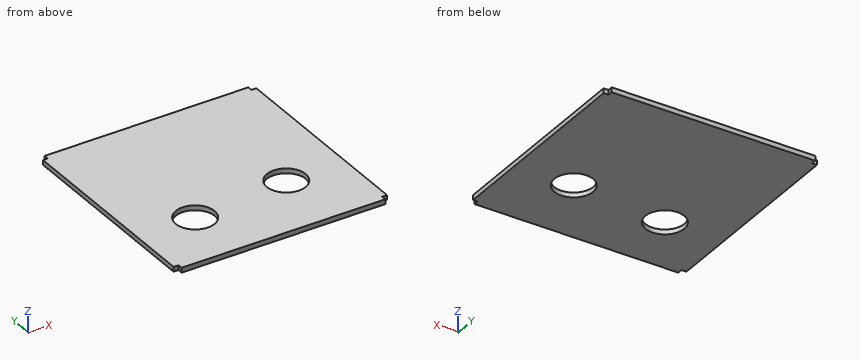
```python
from build123d import *

# Parameters (mm, degrees)
SKETCH1_W           = 279.4
SKETCH1_H           = 279.4
BOSS_EXTRUDE1_DEPTH = 6.35
SKETCH3_R           = 25.4
CUT_EXTRUDE2_DEPTH  = 198.667656687
SKETCH4_W           = 6.35
SKETCH4_H           = 6.35
CUT_EXTRUDE3_DEPTH  = 198.667656687


with BuildPart() as part:
    # Sketch1 → Boss-Extrude1 (new body)
    with BuildSketch(Plane.XY):
        Rectangle(SKETCH1_W, SKETCH1_H)
    extrude(amount=BOSS_EXTRUDE1_DEPTH)

    # Sketch3 → Cut-Extrude2 (cut, through all)
    with BuildSketch(Plane.XY.offset(6.35)):
        with Locations((-63.668986787, -58.7375)):
            Circle(SKETCH3_R)
        with Locations((62.797291543, -47.625)):
            Circle(SKETCH3_R)
    extrude(amount=-CUT_EXTRUDE2_DEPTH, mode=Mode.SUBTRACT)

    # Sketch4 → Cut-Extrude3 (cut, through all)
    with BuildSketch(Plane.XY.offset(6.35)):
        with Locations((-136.525, 136.525)):
            Rectangle(SKETCH4_W, SKETCH4_H)
        with Locations((136.525, 136.525)):
            Rectangle(SKETCH4_W, SKETCH4_H)
        with Locations((136.525, -136.525)):
            Rectangle(SKETCH4_W, SKETCH4_H)
        with Locations((-136.525, -136.525)):
            Rectangle(SKETCH4_W, SKETCH4_H)
    extrude(amount=-CUT_EXTRUDE3_DEPTH, mode=Mode.SUBTRACT)


solid = part.part
```
Part model, mm, in its own coordinate system. Coordinates: 2 decimals unless noted, no trailing zeros. Write each loop counter-clockwise with the first axis right and the second up, starting at its lowest first coordinate (ties: lowest second). Pieces come first, ordered by that corner, then holes.
Item 1: Pin check, flat tips, straight feed: pin 1 (1.9 mm diameter, centred on x = -135, z = 2.5, fed in from +Y); pin 2 (1.9 mm diameter, centred on y = -136, z = 3, fed in from +X); pin 3 (3 mm diameter, centred on y = -136, z = 3, fed in from -X). Stop position of each tip, or through.
Item 2: Probe line 1 (X direction, y = -63.5, z = 5.25); line 2 (X direction, y = -65, z = 3.75); line 3 (X direction, y = -29, z = 3.25). List the from-to ranges inside material, lowest first.
Item 3: Slice it at A-A (x = 52.5). Write the cut outline in (y, z), and give its area (3 significant figures).
Item 4: Slice it at D-D (x = -85). Write the cut outline in (y, z), and give its area (3 significant figures).
Item 5: Slice it at B-B (y = -52.5). Write the cut outline in (x, z).
Item 6: Slice it at C-C (z = 4.5). Count the separate pieces of the cut face and the enclosed holes in it, and give its area (3 significant figures).
Results found:
1. pin 1: stops at y = 133.35
1. pin 2: stops at x = 133.35
1. pin 3: stops at x = -133.35
2. line 1: x = -139.7 to -88.62, -38.72 to 42.97, 82.63 to 139.7
2. line 2: x = -139.7 to -88.28, -39.05 to 44.27, 81.32 to 139.7
2. line 3: x = -139.7 to 45.53, 80.07 to 139.7
3. outline: (-139.7, 0) - (-70.84, 0) - (-70.84, 6.35) - (-139.7, 6.35) - close; (-24.41, 0) - (139.7, 0) - (139.7, 6.35) - (-24.41, 6.35) - close
3. area: 1,480 mm2
4. outline: (-139.7, 0) - (-72.53, 0) - (-72.53, 6.35) - (-139.7, 6.35) - close; (-44.95, 0) - (139.7, 0) - (139.7, 6.35) - (-44.95, 6.35) - close
4. area: 1,600 mm2
5. outline: (-139.7, 0) - (-88.29, 0) - (-88.29, 6.35) - (-139.7, 6.35) - close; (-39.05, 0) - (37.87, 0) - (37.87, 6.35) - (-39.05, 6.35) - close; (87.73, 0) - (139.7, 0) - (139.7, 6.35) - (87.73, 6.35) - close
6. separate pieces: 1
6. enclosed holes: 2
6. area: 73,800 mm2
